Design review of the part built by this model. Coordinates are the model's own, in mm. A direction names the side the tool comes from. Coordinates: 2 decimals unless noted, no trailing zeros. Write each loop counter-clockwise with the first axis right and the second up, starting at its lowest first coordinate (ties: lowest second). Pieces come first, ordered by that corner, then holes. Notation, with made-up numbers: (-24.5, 19) - (-14.5, 19) arc R25 cw to (-14.5, 40) - close; hole circle Ø8 at (24.5, -25.5). An arc over 180 degrees is marked (long way). Answer as CSV lines item,"result". Start each with the question number.
Q1. Clearance check with flat-ended pins moving along their axes: pin 1 (6 mm diameter, centred on x = 0.5, y = -111, fed in from +Z); pin 2 (4.5 mm diameter, centred on x = -7, y = 15, fed in from -Z); pin 3 (0.5 mm diameter, centred on y = -137.5, z = -4, fed in from -X); pin 4 (2 mm diameter, centred on x = 0, y = -44, fed in from +Z). State where each tip first meets the part, or that it passes through.
Q2. We need section A-A (z = -5.75). Write out the cut boundary in (x, y).
Q3. Mouldability with a two-part tool opening along Y and no side actions: class faces 6 (the face through (-7, -66, -2.55)), 7 (the face through (-8.75, -28, -2)), 8 (the face through (2, -147.035, -3)), 9 (the face through (-5.9, -69.1, -3.4)) as pulls with the +Y half, pulls with the -Y half, needs draft (parallel to the pull), parting line crosses it, or undercut.
Q4. We need section B-B (y = -2.5). Write out the cut boundary in (x, z).
Q5. Machinability: for faces 1 (the face through (-7, 17, -2.55)), 2 (the face through (-7, -134, -2.55)), 3 (the face through (-5.816, 96.744, -2.095)), 4 (the face through (3, 106.965, -2)), 5 (the face through (-2, -131, -1.7)), which of the approach directions +Z, -Z, +X, -X, +Y, -Y give a long, thin tool a straight path to every point of the face, cutting with its end or side? Answer none if there is none.
Q6. For line 1 along Z through (x, y) = (-3.5, 61); line 2 along X through (y, z) = (92.5, -1.25); line 3 along X through (y, z) = (-115.5, -3.5), list the stretches that pass through material, from the lowest coordinate up. Write a range as [from, to].
from build123d import *

# Parameters (mm, degrees)
F1_DEPTH    = 4.25
F2_W        = 3.9
F2_H        = 25.4
F3_DEPTH    = 1.7
F4_DEPTH    = 3.165
F5_R        = 1
F6_T1_DEPTH = 11.6817943787
F8_DEPTH    = 1.7
F9_DEPTH    = 25


# Not quite as in the source:
# - a fillet or chamfer that OpenCascade refuses, or shapes differently, is made with other operations: its cross-section is extruded or revolved along the edge and cut away or added
# - a feature names something its author has since deleted; it is built from what else it names


with BuildPart() as f1:
    # F0 (on Top) → F1 (new body)
    with BuildSketch(Plane.XY):
        Polygon((8.75, 106.9650896668), (-2.75, 106.9650896668), (-8.75, 86.9647799072), (-8.75, -147.0349103332), (8.75, -147.0349103332), align=None)
    extrude(amount=-F1_DEPTH)

    # F2 (on face) → F3 (cut)
    with BuildSketch(Plane(origin=(0, 0, -4.25), x_dir=(1, 0, 0), z_dir=(0, 0, -1))):
        with Locations((-6.8, 134.3349103332)):
            Rectangle(F2_W, F2_H)
        Polygon((-8.75, 78.5952200928), (-8.75, 58.5949103332), (-2.75, 58.5949103332), align=None)
        Polygon((-8.75, -4.1847799072), (-8.75, -24.1850896668), (-2.75, -24.1850896668), align=None)
    extrude(amount=-F3_DEPTH, mode=Mode.SUBTRACT)

    # F2 (on face) → F4 (join)
    with BuildSketch(Plane(origin=(0, 0, -4.25), x_dir=(1, 0, 0), z_dir=(0, 0, -1))):
        Polygon((2.75, 147.0349103332), (8.75, 127.0349103332), (8.75, 147.0349103332), align=None)
    extrude(amount=F4_DEPTH)

    # F5
    f5_edges = [f1.edges().sort_by_distance(p)[0] for p in [
        (-2.75, -58.59491, -3.4),
        (-8.75, -58.59491, -3.4),
        (-4.85, -121.63491, -3.4),
        (-8.75, -121.63491, -3.4),
        (-4.85, -147.03491, -3.4),
        (-8.75, -147.03491, -1.275),
        (8.75, -147.03491, -3.7075),
        (2.75, -147.03491, -5.8325),
        (-2.75, 24.18509, -3.4),
        (-8.75, 24.18509, -3.4),
        (8.75, 106.96509, -2.125),
        (-2.75, 106.96509, -2.125),
    ]]
    fillet(f5_edges, radius=F5_R)

    # F6: fillet of radius 0.5 on 1 edges, made by hand

    # F6_s2 → F6_t1 (cut)
    with BuildSketch(Plane.XY.offset(-15.9317943787)):
        with BuildLine():
            ThreePointArc((8.75, -130.4416280846), (8.3226065723, -129.9469278869), (7.7710868574, -130.2979541419))
            Line((7.7710868574, -130.2979541419), (8.75, -127.0349103332))
            Line((8.75, -127.0349103332), (8.75, -130.4416280846))
        make_face()
    extrude(amount=F6_T1_DEPTH, mode=Mode.SUBTRACT)

    # F7 (on face) → F8 (cut)
    with BuildSketch(Plane.XY):
        with BuildLine():
            Line((-1.281113759, 101.2524492275), (-3.5080282296, 93.8292860243))
            ThreePointArc((-3.5080282296, 93.8292860243), (-1.8318189791, 90.7163576177), (1.2811093315, 92.3925670464))
            Line((1.2811093315, 92.3925670464), (3.508023802, 99.8157302495))
            ThreePointArc((3.508023802, 99.8157302495), (1.831814489, 102.9286584474), (-1.281113759, 101.2524492275))
        make_face()
        with BuildLine():
            Line((2.5501962221, 100.1030738196), (0.3232817516, 92.6799106164))
            ThreePointArc((0.3232817516, 92.6799106164), (-1.5444751953, 91.6741851335), (-2.5502007779, 93.5419420268))
            Line((-2.5502007779, 93.5419420268), (-0.3232863074, 100.9651052299))
            ThreePointArc((-0.3232863074, 100.9651052299), (1.5444707052, 101.9708309316), (2.5501962221, 100.1030738196))
        make_face(mode=Mode.SUBTRACT)
        with BuildLine():
            Line((-1.281113759, 81.8682859589), (-3.5080282296, 74.4451227557))
            ThreePointArc((-3.5080282296, 74.4451227557), (-1.8318189791, 71.3321943492), (1.2811093315, 73.0084037778))
            Line((1.2811093315, 73.0084037778), (3.508023802, 80.431566981))
            ThreePointArc((3.508023802, 80.431566981), (1.831814489, 83.5444951788), (-1.281113759, 81.8682859589))
        make_face()
        with BuildLine():
            Line((2.5501962221, 80.718910551), (0.3232817516, 73.2957473478))
            ThreePointArc((0.3232817516, 73.2957473478), (-1.5444751953, 72.2900218649), (-2.5502007779, 74.1577787582))
            Line((-2.5502007779, 74.1577787582), (-0.3232863074, 81.5809419614))
            ThreePointArc((-0.3232863074, 81.5809419614), (1.5444707052, 82.586667663), (2.5501962221, 80.718910551))
        make_face(mode=Mode.SUBTRACT)
        with BuildLine():
            Line((-1.3184834487, -37.2262845319), (-3.5453934487, -44.6494328331))
            ThreePointArc((-3.5453934487, -44.6494328331), (-1.6928299922, -47.6607462741), (1.3184834487, -45.8081828176))
            Line((1.3184834487, -45.8081828176), (3.5453934487, -38.3850345164))
            ThreePointArc((3.5453934487, -38.3850345164), (1.6928299922, -35.3737210755), (-1.3184834487, -37.2262845319))
        make_face()
        with BuildLine():
            ThreePointArc((-0.32342291, -37.3750995728), (1.5027069877, -36.3570453968), (2.5726180692, -38.1532845195))
            Line((2.5726180692, -38.1532845195), (0.3457080692, -45.5764328207))
            ThreePointArc((0.3457080692, -45.5764328207), (-1.4610799953, -46.6879708946), (-2.5726180692, -44.88118283))
            Line((-2.5726180692, -44.88118283), (-0.32342291, -37.3750995728))
        make_face(mode=Mode.SUBTRACT)
        with BuildLine():
            ThreePointArc((-3.5453934487, -25.2652845319), (-1.6928299922, -28.2765979729), (1.3184834487, -26.4240345164))
            Line((1.3184834487, -26.4240345164), (3.5453979193, -19.0008713133))
            ThreePointArc((3.5453979193, -19.0008713133), (1.6928344628, -15.9895578723), (-1.3184789782, -17.8421213288))
            Line((-1.3184789782, -17.8421213288), (-3.5453934487, -25.2652845319))
        make_face()
        with BuildLine():
            ThreePointArc((0.3513294529, -26.167779481), (-1.4365749568, -27.3094439771), (-2.5782394529, -25.5215395674))
            Line((-2.5782394529, -25.5215395674), (-0.3513249813, -18.0983763605))
            ThreePointArc((-0.3513249813, -18.0983763605), (1.4365749587, -16.9567321352), (2.5782439235, -18.7446162778))
            Line((2.5782439235, -18.7446162778), (0.3513294529, -26.167779481))
        make_face(mode=Mode.SUBTRACT)
        with BuildLine():
            Line((-1.2811093046, -107.9180212426), (-3.5080237752, -115.3411844458))
            ThreePointArc((-3.5080237752, -115.3411844458), (-1.8318145066, -118.4541127276), (1.2811137752, -116.7779034591))
            Line((1.2811137752, -116.7779034591), (3.5080282457, -109.3547402559))
            ThreePointArc((3.5080282457, -109.3547402559), (1.8318145067, -106.2418268761), (-1.2811093046, -107.9180212426))
        make_face()
        with BuildLine():
            ThreePointArc((-0.3232817945, -108.2053650453), (1.544470704, -107.1996543861), (2.5502007356, -109.0673964532))
            Line((2.5502007356, -109.0673964532), (0.3232862651, -116.4905596564))
            ThreePointArc((0.3232862651, -116.4905596564), (-1.544470704, -117.4962852176), (-2.5501962651, -115.6285282484))
            Line((-2.5501962651, -115.6285282484), (-0.3232817945, -108.2053650453))
        make_face(mode=Mode.SUBTRACT)
        with BuildLine():
            Line((-1.280113287, -127.2988486416), (-3.507023287, -134.7220131859))
            ThreePointArc((-3.507023287, -134.7220131859), (-1.8036595485, -137.8465346478), (1.2982333531, -136.1023033504))
            Line((1.2982333531, -136.1023033504), (3.5251433531, -128.6791388061))
            ThreePointArc((3.5251433531, -128.6791388061), (1.8036595485, -125.6176994193), (-1.280113287, -127.2988486416))
        make_face()
        with BuildLine():
            ThreePointArc((0.308713365, -135.9206030083), (-1.5472756815, -136.8795961043), (-2.5617754063, -135.0533558662))
            Line((-2.5617754063, -135.0533558662), (-0.3348654063, -127.6301913219))
            ThreePointArc((-0.3348654063, -127.6301913219), (1.5472756815, -126.5846379628), (2.535623365, -128.4974384639))
            Line((2.535623365, -128.4974384639), (0.308713365, -135.9206030083))
        make_face(mode=Mode.SUBTRACT)
    extrude(amount=-F8_DEPTH, mode=Mode.SUBTRACT)

    # F7 (on face) → F9 (cut)
    with BuildSketch(Plane.XY):
        with BuildLine():
            Line((-0.3348654063, -127.6301913219), (-2.5617754063, -135.0533558662))
            ThreePointArc((-2.5617754063, -135.0533558662), (-1.5472756815, -136.8795961043), (0.308713365, -135.9206030083))
            Line((0.308713365, -135.9206030083), (2.535623365, -128.4974384639))
            ThreePointArc((2.535623365, -128.4974384639), (1.5472756815, -126.5846379628), (-0.3348654063, -127.6301913219))
        make_face()
        with BuildLine():
            Line((0.3232862651, -116.4905596564), (2.5502007356, -109.0673964532))
            ThreePointArc((2.5502007356, -109.0673964532), (1.544470704, -107.1996543861), (-0.3232817945, -108.2053650453))
            Line((-0.3232817945, -108.2053650453), (-2.5501962651, -115.6285282484))
            ThreePointArc((-2.5501962651, -115.6285282484), (-1.544470704, -117.4962852176), (0.3232862651, -116.4905596564))
        make_face()
        with BuildLine():
            Line((0.3457080692, -45.5764328207), (2.5726180692, -38.1532845195))
            ThreePointArc((2.5726180692, -38.1532845195), (1.5027069877, -36.3570453968), (-0.32342291, -37.3750995728))
            Line((-0.32342291, -37.3750995728), (-2.5726180692, -44.88118283))
            ThreePointArc((-2.5726180692, -44.88118283), (-1.4610799953, -46.6879708946), (0.3457080692, -45.5764328207))
        make_face()
        with BuildLine():
            Line((-0.3513249813, -18.0983763605), (-2.5782394529, -25.5215395674))
            ThreePointArc((-2.5782394529, -25.5215395674), (-1.4365749568, -27.3094439771), (0.3513294529, -26.167779481))
            Line((0.3513294529, -26.167779481), (2.5782439235, -18.7446162778))
            ThreePointArc((2.5782439235, -18.7446162778), (1.4365749587, -16.9567321352), (-0.3513249813, -18.0983763605))
        make_face()
        with BuildLine():
            ThreePointArc((-2.5502007779, 93.5419420268), (-1.5444751953, 91.6741851335), (0.3232817516, 92.6799106164))
            Line((0.3232817516, 92.6799106164), (2.5501962221, 100.1030738196))
            ThreePointArc((2.5501962221, 100.1030738196), (1.5444707052, 101.9708309316), (-0.3232863074, 100.9651052299))
            Line((-0.3232863074, 100.9651052299), (-2.5502007779, 93.5419420268))
        make_face()
        with BuildLine():
            ThreePointArc((-2.5502007779, 74.1577787582), (-1.5444751953, 72.2900218649), (0.3232817516, 73.2957473478))
            Line((0.3232817516, 73.2957473478), (2.5501962221, 80.718910551))
            ThreePointArc((2.5501962221, 80.718910551), (1.5444707052, 82.586667663), (-0.3232863074, 81.5809419614))
            Line((-0.3232863074, 81.5809419614), (-2.5502007779, 74.1577787582))
        make_face()
    extrude(amount=-F9_DEPTH, mode=Mode.SUBTRACT)


solid = f1.part
Results list:
1,pin 1,"stops at z = 0"
1,pin 2,"stops at z = -4.25"
1,pin 3,"stops at x = -4.85"
1,pin 4,"stops at z = -1.7"
2,outline,"(3.14, -145.75) arc R1 ccw to (4.09, -147.03) - (7.75, -147.03) arc R1 ccw to (8.75, -146.03) - (8.75, -130.44) arc R0.5 ccw to (7.77, -130.3) - close"
3,face 6,"undercut"
3,face 7,"needs draft"
3,face 8,"pulls with the -Y half"
3,face 9,"undercut"
4,outline,"(-8.75, -4.25) - (8.75, -4.25) - (8.75, 0) - (-8.75, 0) - close"
5,face 1,"-Z, -X"
5,face 2,"-Z, -X, -Y"
5,face 3,"+Z, -Z, -X, +Y"
5,face 4,"+Z, -Z, +X, -X, +Y"
5,face 5,"+Z"
6,line 1,"z = [-4.25, 0]"
6,line 2,"x = [-7.09, -3.54], [1.31, 8.75]"
6,line 3,"x = [-8.75, -2.51], [0.62, 8.75]"
